Could you check a few things on this model? Use its own coordinates, in mm. A direction names the side the tool comes from. Round coordinates to 2 decimals unless told otherwise and drop trailing zeros. Write each loop counter-clockwise with the first axis right and the second up, starting at its lowest first coordinate (ties: lowest second). Pieces come first, ordered by that corner, then holes. Notation, with made-up numbers: (-39.5, 34) -> (-7.5, 34) arc R29 ccw to (-7.5, 64) -> close; hole circle Ø4 at (55.5, 27). An arc over 180 degrees is marked (long way). One line per question, with ' | ' between items. Start each with the question number.
1. Imagine slicing it at B-B, the plane y = -13.5. List the corners of the cut face in (x, z) for me, and give its area (3 significant figures).
2. Imagine slicing it at A-A, the plane z = -241. List the corners of the cut face in (x, y) for me.
3. For faces 4 (the flat face through (4.8, 1, 6)), 5 (the flat face through (20, -54, 450)), which set-ups out of +Z, -Z, +X, -X, +Y, -Y let a thin tool reach every point of the face, with its end or its side?
4. If I drill on line 1 along Y through (x, z) = (29.5, 89); line 2 along X through (y, z) = (-56.5, 0); line 3 along X through (y, z) = (-43, 32), over which ranges is the centre line in solid material (lowest first)? Write a range as [from, to].
5. Thinking about a two-plate mould opening in Y: for faces 1 (the flat face through (26.4, -60, 6.3)), 2 (the flat face through (3, 0, -450)), 3 (the cylindrical face through (2.366, -0.495, 392.505)), which applies, released by +Y, released by -Y, zero draft, split by the parting line, or undercut?
6. For pin 1 Ø10 at (x, z) = (26.55, 0) entering from -Y; pin 2 Ø6 at (y, z) = (-42, -341.5) entering from +X, each with a flat end and sliding along its axis, tell me the tip position at first contact or that it passes through.
from build123d import *

# Parameters (mm, degrees)
EXTRUDE_1_DEPTH          = 450
CUT_EXTRUDE_1_DEPTH      = 5
FILLET_1_R               = 10
CUT_EXTRUDE_2_DEPTH      = 469.619248431
CUT_EXTRUDE_2_DEPTH_BACK = 469.619248431
SKETCH_3_R               = 6.1


with BuildPart() as part:
    # Эскиз1 → Бобышка-Вытянуть1 (new, symmetric)
    with BuildSketch(Plane.XY):
        with BuildLine():
            Line((0, -60), (0, 60))
            Line((0, 60), (52, 60))
            Line((52, 60), (52, 56.7))
            ThreePointArc((52, 56.7), (50.681980515, 53.518019485), (47.5, 52.2))
            Line((47.5, 52.2), (12.3, 52.2))
            ThreePointArc((12.3, 52.2), (6.996699141, 50.003300859), (4.8, 44.7))
            Line((4.8, 44.7), (4.8, -44.7))
            ThreePointArc((4.8, -44.7), (6.996699141, -50.003300859), (12.3, -52.2))
            Line((12.3, -52.2), (47.5, -52.2))
            ThreePointArc((47.5, -52.2), (50.681980515, -53.518019485), (52, -56.7))
            Line((52, -56.7), (52, -60))
            Line((52, -60), (0, -60))
        make_face()
    extrude(amount=EXTRUDE_1_DEPTH, both=True)

    # Эскиз2 → Вырез-Вытянуть1 (cut, symmetric)
    with BuildSketch(Plane.ZY):
        with BuildLine():
            Line((415, 22.5), (450, 22.5))
            Line((450, 22.5), (450, -22.5))
            Line((450, -22.5), (415, -22.5))
            ThreePointArc((415, -22.5), (392.5, 0), (415, 22.5))
        make_face()
    extrude(amount=CUT_EXTRUDE_1_DEPTH, both=True, mode=Mode.SUBTRACT)

    # Скругление1
    fillet_1_edges = [part.edges().sort_by_distance(p)[0] for p in [
        (2.4, -22.5, 450),
        (2.4, 22.5, 450),
    ]]
    fillet(fillet_1_edges, radius=FILLET_1_R)

    # Эскиз3 → Вырез-Вытянуть2 (cut, two sides: drawn at the far end of the back side and taken through both)
    with BuildSketch(Plane(origin=(0, 60, 0), x_dir=(1, 0, 0), z_dir=(0, 1, 0)).offset(-CUT_EXTRUDE_2_DEPTH_BACK)):
        with Locations(Location((26.550751723, -300, 0), (0, 0, 180))):
            Circle(SKETCH_3_R)
        with Locations(Location((26.550751723, -200, 0), (0, 0, 180))):
            Circle(SKETCH_3_R)
        with Locations(Location((26.550751723, -100, 0), (0, 0, 180))):
            Circle(SKETCH_3_R)
        with Locations(Location((26.550751723, 0, 0), (0, 0, 180))):
            Circle(SKETCH_3_R)
        with Locations(Location((26.550751723, 100, 0), (0, 0, 180))):
            Circle(SKETCH_3_R)
    extrude(amount=CUT_EXTRUDE_2_DEPTH + CUT_EXTRUDE_2_DEPTH_BACK, mode=Mode.SUBTRACT)


solid = part.part
Geometry results:
1) outline: (0, -450) -> (4.8, -450) -> (4.8, 397) -> (0, 397) -> close | area: 4,070 mm2
2) outline: (0, -60) -> (52, -60) -> (52, -56.7) arc R4.5 ccw to (47.5, -52.2) -> (12.3, -52.2) arc R7.5 cw to (4.8, -44.7) -> (4.8, 44.7) arc R7.5 cw to (12.3, 52.2) -> (47.5, 52.2) arc R4.5 ccw to (52, 56.7) -> (52, 60) -> (0, 60) -> close
3) face 4: +Z, -Z, +X | face 5: +Z, +X, -X, +Y, -Y
4) line 1: y = [-60, -52.2], [52.2, 60] | line 2: x = [0, 20.45], [32.65, 52] | line 3: x = [0, 4.8]
5) face 1: released by -Y | face 2: zero draft | face 3: undercut
6) pin 1: passes through | pin 2: stops at x = 4.81
